```python
from build123d import *
from build123d.topology import SkipClean

# Parameters (mm, degrees)
SKETCH1_R           = 2.1
BOSS_EXTRUDE1_DEPTH = 350
SKETCH3_R           = 2.75
CUT_EXTRUDE1_DEPTH  = 10
SKETCH4_R           = 2.1
BOSS_EXTRUDE2_DEPTH = 50


with BuildPart() as part:
    # Sketch1 → Boss-Extrude1 (new body)
    with BuildSketch(Plane.XY):
        with BuildLine():
            Line((-8, 4), (-8, 7))
            Line((-8, 7), (-10, 7))
            Line((-10, 7), (-10, -7))
            Line((-10, -7), (-8, -7))
            Line((-8, -7), (-8, -4))
            Line((-8, -4), (-7.060660172, -4))
            Line((-7.060660172, -4), (-4, -7.060660172))
            Line((-4, -7.060660172), (-4, -9.480384758))
            Line((-4, -9.480384758), (-3.7, -10))
            Line((-3.7, -10), (-4, -10.519615242))
            Line((-4, -10.519615242), (-4, -12.939339828))
            Line((-4, -12.939339828), (-7.060660172, -16))
            Line((-7.060660172, -16), (-8, -16))
            Line((-8, -16), (-8, -13))
            Line((-8, -13), (-10, -13))
            Line((-10, -13), (-10, -19))
            ThreePointArc((-10, -19), (-9.707106781, -19.707106781), (-9, -20))
            Line((-9, -20), (-3, -20))
            Line((-3, -20), (-3, -18))
            Line((-3, -18), (-6, -18))
            Line((-6, -18), (-6, -17.060660172))
            Line((-6, -17.060660172), (-2.939339828, -14))
            Line((-2.939339828, -14), (-0.519615242, -14))
            Line((-0.519615242, -14), (0, -13.7))
            Line((0, -13.7), (0.519615242, -14))
            Line((0.519615242, -14), (2.939339828, -14))
            Line((2.939339828, -14), (6, -17.060660172))
            Line((6, -17.060660172), (6, -18))
            Line((6, -18), (3, -18))
            Line((3, -18), (3, -20))
            Line((3, -20), (9, -20))
            ThreePointArc((9, -20), (9.707106781, -19.707106781), (10, -19))
            Line((10, -19), (10, -13))
            Line((10, -13), (8, -13))
            Line((8, -13), (8, -16))
            Line((8, -16), (7.060660172, -16))
            Line((7.060660172, -16), (4, -12.939339828))
            Line((4, -12.939339828), (4, -10.519615242))
            Line((4, -10.519615242), (3.7, -10))
            Line((3.7, -10), (4, -9.480384758))
            Line((4, -9.480384758), (4, -7.060660172))
            Line((4, -7.060660172), (7.060660172, -4))
            Line((7.060660172, -4), (8, -4))
            Line((8, -4), (8, -7))
            Line((8, -7), (10, -7))
            Line((10, -7), (10, 7))
            Line((10, 7), (8, 7))
            Line((8, 7), (8, 4))
            Line((8, 4), (7.060660172, 4))
            Line((7.060660172, 4), (4, 7.060660172))
            Line((4, 7.060660172), (4, 9.480384758))
            Line((4, 9.480384758), (3.7, 10))
            Line((3.7, 10), (4, 10.519615242))
            Line((4, 10.519615242), (4, 12.939339828))
            Line((4, 12.939339828), (7.060660172, 16))
            Line((7.060660172, 16), (8, 16))
            Line((8, 16), (8, 13))
            Line((8, 13), (10, 13))
            Line((10, 13), (10, 19))
            ThreePointArc((10, 19), (9.707106781, 19.707106781), (9, 20))
            Line((9, 20), (3, 20))
            Line((3, 20), (3, 18))
            Line((3, 18), (6, 18))
            Line((6, 18), (6, 17.060660172))
            Line((6, 17.060660172), (2.939339828, 14))
            Line((2.939339828, 14), (0.519615242, 14))
            Line((0.519615242, 14), (0, 13.7))
            Line((0, 13.7), (-0.519615242, 14))
            Line((-0.519615242, 14), (-2.939339828, 14))
            Line((-2.939339828, 14), (-6, 17.060660172))
            Line((-6, 17.060660172), (-6, 18))
            Line((-6, 18), (-3, 18))
            Line((-3, 18), (-3, 20))
            Line((-3, 20), (-9, 20))
            ThreePointArc((-9, 20), (-9.707106781, 19.707106781), (-10, 19))
            Line((-10, 19), (-10, 13))
            Line((-10, 13), (-8, 13))
            Line((-8, 13), (-8, 16))
            Line((-8, 16), (-7.060660172, 16))
            Line((-7.060660172, 16), (-4, 12.939339828))
            Line((-4, 12.939339828), (-4, 10.519615242))
            Line((-4, 10.519615242), (-3.7, 10))
            Line((-3.7, 10), (-4, 9.480384758))
            Line((-4, 9.480384758), (-4, 7.060660172))
            Line((-4, 7.060660172), (-7.060660172, 4))
            Line((-7.060660172, 4), (-8, 4))
        make_face()
        with Locations(Location((0, 10, 0), (0, 0, 180))):
            Circle(SKETCH1_R, mode=Mode.SUBTRACT)
        with Locations(Location((0, -10, 0), (0, 0, 180))):
            Circle(SKETCH1_R, mode=Mode.SUBTRACT)
        with BuildLine():
            Line((-8, -1.7), (-8, 1.7))
            ThreePointArc((-8, 1.7), (-7.912132034, 1.912132034), (-7.7, 2))
            Line((-7.7, 2), (-7.063603897, 2))
            ThreePointArc((-7.063603897, 2), (-6.948798867, 2.02283614), (-6.851471863, 2.087867966))
            Line((-6.851471863, 2.087867966), (-2.939339828, 6))
            Line((-2.939339828, 6), (2.939339828, 6))
            Line((2.939339828, 6), (6.851471863, 2.087867966))
            ThreePointArc((6.851471863, 2.087867966), (6.948798867, 2.02283614), (7.063603897, 2))
            Line((7.063603897, 2), (7.7, 2))
            ThreePointArc((7.7, 2), (7.912132034, 1.912132034), (8, 1.7))
            Line((8, 1.7), (8, -1.7))
            ThreePointArc((8, -1.7), (7.912132034, -1.912132034), (7.7, -2))
            Line((7.7, -2), (7.063603897, -2))
            ThreePointArc((7.063603897, -2), (6.948798867, -2.02283614), (6.851471863, -2.087867966))
            Line((6.851471863, -2.087867966), (2.939339828, -6))
            Line((2.939339828, -6), (-2.939339828, -6))
            Line((-2.939339828, -6), (-6.851471863, -2.087867966))
            ThreePointArc((-6.851471863, -2.087867966), (-6.948798867, -2.02283614), (-7.063603897, -2))
            Line((-7.063603897, -2), (-7.7, -2))
            ThreePointArc((-7.7, -2), (-7.912132034, -1.912132034), (-8, -1.7))
        make_face(mode=Mode.SUBTRACT)
    extrude(amount=-BOSS_EXTRUDE1_DEPTH)

    # Sketch3 → Cut-Extrude1 (cut)
    with BuildSketch(Plane.XZ.offset(14)):
        with Locations(Location((0, -9, 0), (0, 0, 270))):
            Circle(SKETCH3_R)
    extrude(amount=-CUT_EXTRUDE1_DEPTH, mode=Mode.SUBTRACT)

    # Sketch4 → Boss-Extrude2 (add)
    with SkipClean():  # the faces are left unmerged after this step: merging them gives an invalid solid
        with BuildSketch(Plane(origin=(0, 0, -350), x_dir=(-1, 0, 0), z_dir=(0, 0, -1))):
            with BuildLine():
                Line((8, 4), (7.060660172, 4))
                Line((7.060660172, 4), (4, 7.060660172))
                Line((4, 7.060660172), (4, 9.480384758))
                Line((4, 9.480384758), (3.7, 10))
                Line((3.7, 10), (4, 10.519615242))
                Line((4, 10.519615242), (4, 12.939339828))
                Line((4, 12.939339828), (7.060660172, 16))
                Line((7.060660172, 16), (8, 16))
                Line((8, 16), (8, 13))
                Line((8, 13), (10, 13))
                Line((10, 13), (10, 19))
                ThreePointArc((10, 19), (9.707106781, 19.707106781), (9, 20))
                Line((9, 20), (3, 20))
                Line((3, 20), (3, 18))
                Line((3, 18), (6, 18))
                Line((6, 18), (6, 17.060660172))
                Line((6, 17.060660172), (2.939339828, 14))
                Line((2.939339828, 14), (0.519615242, 14))
                Line((0.519615242, 14), (0, 13.7))
                Line((0, 13.7), (-0.519615242, 14))
                Line((-0.519615242, 14), (-2.939339828, 14))
                Line((-2.939339828, 14), (-6, 17.060660172))
                Line((-6, 17.060660172), (-6, 18))
                Line((-6, 18), (-3, 18))
                Line((-3, 18), (-3, 20))
                Line((-3, 20), (-9, 20))
                ThreePointArc((-9, 20), (-9.707106781, 19.707106781), (-10, 19))
                Line((-10, 19), (-10, 13))
                Line((-10, 13), (-8, 13))
                Line((-8, 13), (-8, 16))
                Line((-8, 16), (-7.060660172, 16))
                Line((-7.060660172, 16), (-4, 12.939339828))
                Line((-4, 12.939339828), (-4, 10.519615242))
                Line((-4, 10.519615242), (-3.7, 10))
                Line((-3.7, 10), (-4, 9.480384758))
                Line((-4, 9.480384758), (-4, 7.060660172))
                Line((-4, 7.060660172), (-7.060660172, 4))
                Line((-7.060660172, 4), (-8, 4))
                Line((-8, 4), (-8, 7))
                Line((-8, 7), (-10, 7))
                Line((-10, 7), (-10, -7))
                Line((-10, -7), (-8, -7))
                Line((-8, -7), (-8, -4))
                Line((-8, -4), (-7.060660172, -4))
                Line((-7.060660172, -4), (-4, -7.060660172))
                Line((-4, -7.060660172), (-4, -9.480384758))
                Line((-4, -9.480384758), (-3.7, -10))
                Line((-3.7, -10), (-4, -10.519615242))
                Line((-4, -10.519615242), (-4, -12.939339828))
                Line((-4, -12.939339828), (-7.060660172, -16))
                Line((-7.060660172, -16), (-8, -16))
                Line((-8, -16), (-8, -13))
                Line((-8, -13), (-10, -13))
                Line((-10, -13), (-10, -19))
                ThreePointArc((-10, -19), (-9.707106781, -19.707106781), (-9, -20))
                Line((-9, -20), (-3, -20))
                Line((-3, -20), (-3, -18))
                Line((-3, -18), (-6, -18))
                Line((-6, -18), (-6, -17.060660172))
                Line((-6, -17.060660172), (-2.939339828, -14))
                Line((-2.939339828, -14), (-0.519615242, -14))
                Line((-0.519615242, -14), (0, -13.7))
                Line((0, -13.7), (0.519615242, -14))
                Line((0.519615242, -14), (2.939339828, -14))
                Line((2.939339828, -14), (6, -17.060660172))
                Line((6, -17.060660172), (6, -18))
                Line((6, -18), (3, -18))
                Line((3, -18), (3, -20))
                Line((3, -20), (9, -20))
                ThreePointArc((9, -20), (9.707106781, -19.707106781), (10, -19))
                Line((10, -19), (10, -13))
                Line((10, -13), (8, -13))
                Line((8, -13), (8, -16))
                Line((8, -16), (7.060660172, -16))
                Line((7.060660172, -16), (4, -12.939339828))
                Line((4, -12.939339828), (4, -10.519615242))
                Line((4, -10.519615242), (3.7, -10))
                Line((3.7, -10), (4, -9.480384758))
                Line((4, -9.480384758), (4, -7.060660172))
                Line((4, -7.060660172), (7.060660172, -4))
                Line((7.060660172, -4), (8, -4))
                Line((8, -4), (8, -7))
                Line((8, -7), (10, -7))
                Line((10, -7), (10, 7))
                Line((10, 7), (8, 7))
                Line((8, 7), (8, 4))
            make_face()
            with Locations((0, 10)):
                Circle(SKETCH4_R, mode=Mode.SUBTRACT)
            with Locations(Location((0, -10, 0), (0, 0, 180))):
                Circle(SKETCH4_R, mode=Mode.SUBTRACT)
            with BuildLine():
                Line((-2.939339828, 6), (2.939339828, 6))
                Line((2.939339828, 6), (6.851471863, 2.087867966))
                ThreePointArc((6.851471863, 2.087867966), (6.948798867, 2.02283614), (7.063603897, 2))
                Line((7.063603897, 2), (7.7, 2))
                ThreePointArc((7.7, 2), (7.912132034, 1.912132034), (8, 1.7))
                Line((8, 1.7), (8, -1.7))
                ThreePointArc((8, -1.7), (7.912132034, -1.912132034), (7.7, -2))
                Line((7.7, -2), (7.063603897, -2))
                ThreePointArc((7.063603897, -2), (6.948798867, -2.02283614), (6.851471863, -2.087867966))
                Line((6.851471863, -2.087867966), (2.939339828, -6))
                Line((2.939339828, -6), (-2.939339828, -6))
                Line((-2.939339828, -6), (-6.851471863, -2.087867966))
                ThreePointArc((-6.851471863, -2.087867966), (-6.948798867, -2.02283614), (-7.063603897, -2))
                Line((-7.063603897, -2), (-7.7, -2))
                ThreePointArc((-7.7, -2), (-7.912132034, -1.912132034), (-8, -1.7))
                Line((-8, -1.7), (-8, 1.7))
                ThreePointArc((-8, 1.7), (-7.912132034, 1.912132034), (-7.7, 2))
                Line((-7.7, 2), (-7.063603897, 2))
                ThreePointArc((-7.063603897, 2), (-6.948798867, 2.02283614), (-6.851471863, 2.087867966))
                Line((-6.851471863, 2.087867966), (-2.939339828, 6))
            make_face(mode=Mode.SUBTRACT)
        extrude(amount=BOSS_EXTRUDE2_DEPTH)
    add(part.part.scale(1), mode=Mode.REPLACE)  # the faces are merged on a copy


solid = part.part
```
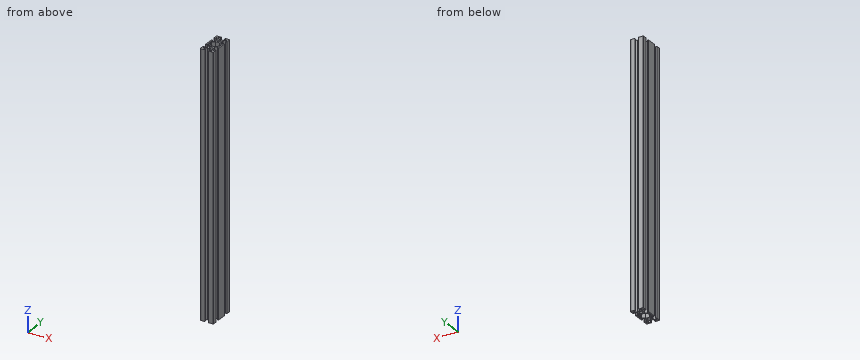
CAD build for the part. Positions are in the model's coordinates, mm. Give positions to 0.01 mm unless a question says otherwise; leave off trailing zeros.
(1) Saw through at A-A, the plane z = -203. State how many separate pieces and enclosed holes the cut face has, then the cut area to 3 significant figures.
(2) Flat gauge pins, fed straight in: pin 1 (1.9 mm diameter, centred on x = 1.5, z = -213.5, fed in from -Y); pin 2 (1.9 mm diameter, centred on y = -11.5, z = -110, fed in from -X). Where does each tip first touch, or does it go through?
(3) Drill centre lines: L1, parallel to Y at x = -8.75, z = -28.5; L2, parallel to Y at x = 0, z = -76; L3, parallel to Y at x = 7.5, z = -35. Where is each one in solid material? Low to high.
Results found:
1. separate pieces: 1
1. enclosed holes: 3
1. area: 324 mm2
2. pin 1: stops at y = -14
2. pin 2: stops at x = -4
3. L1: y = -20 to -13, -7 to 7, 13 to 20
3. L2: y = -13.7 to -12.1, -7.9 to -6, 6 to 7.9, 12.1 to 13.7
3. L3: y = -20 to -16, -4 to -2, 2 to 4, 16 to 20
